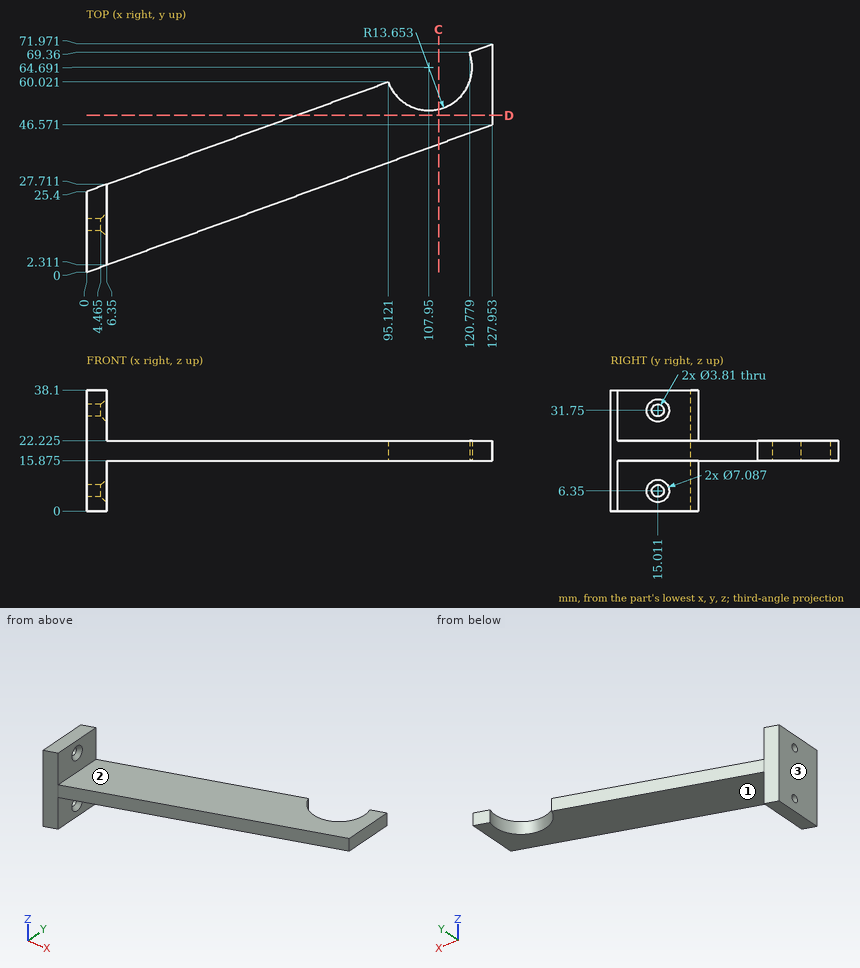
Geometry check sheet. Reference: drawing and pictorial views, mm from the part's lowest x, y, z. A direction names the side the tool comes from. Round coordinates to 2 decimals unless told otherwise and drop trailing zeros. Loops run counter-clockwise (first coordinate to the right, second up) from the corner with the lowest first, then second, coordinate; pieces in that order, holes last. Notation, with made-up numbers: (71.25, -0.5) - (94.25, -0.5) arc R15 ccw to (94.25, 14.5) - close; hole circle Ø5 at (21.5, -35). An arc over 180 degrees is marked (long way). Answer as CSV lines item,"result".
(1) Material ranges on line 1 along X through (y, z) = (23.5, 36); line 2 along Z through (x, y) = (66.5, 25.5) (1 decimal); line 3 along Y through (x, z) = (2, 6) (1 decimal), recorded low to high.
Output values:
line 1,"x = 0 to 6.35"
line 2,"z = 15.9 to 22.2"
line 3,"y = 0.7 to 13.1, 16.9 to 26.1"
(2) Cross-section at C-C, the plane x = 111. Enter the section's corners in (y, z) (1 decimal).
Output values:
outline,"(40.4, 15.9) - (51.4, 15.9) - (51.4, 22.2) - (40.4, 22.2) - close"
(3) Depth check by flat-ended pin: pin 1 Ø6 at (x, z) = (100, 23) entering from -Y; pin 2 Ø2 at (y, z) = (29.5, 32) entering from -X; pin 3 Ø4 at (x, y) = (69, 26.5) entering from +Z (1 decimal); pin 4 Ø5 at (x, y) = (29.5, 36.5) entering from -Z (1 decimal). Enter the tip coordinate at first touch or a pass-through.
Output values:
pin 1,"stops at y = 35.34"
pin 2,"passes through"
pin 3,"stops at z = 22.2"
pin 4,"stops at z = 15.9"
(4) Set-up check for the marked faces 1, 2 and 3: record each of +Z, -Z, +X, -X, +Y, -Y from which the full face is reachable in a straight line by a thin tool's end or side.
Output values:
face 1,"-Z, +X, +Y, -Y"
face 2,"+Z, +X, +Y, -Y"
face 3,"+Z, -Z, -X, +Y, -Y"
(5) Cross-section at D-D, the plane y = 49.5. Enter the section's corners in (x, z) (1 decimal), and give its area (3 significant figures).
Output values:
outline,"(66.2, 15.9) - (128, 15.9) - (128, 22.2) - (66.2, 22.2) - close"
area,"392 mm²"
